Answer from the drawing. Dimensions are ordinates in mm from the lowest x, y and z of the part. A direction names the side the tool comes from. Give positions to 0.01 mm unless a question says otherwise; leave off trailing zeros. Loops run counter-clockwise (first coordinate to the right, second up) from the corner with the lowest first, then second, coordinate; pieces in that order, holes last. Notation, with made-up numbers: M 1,-24.75 L 13,-24.75 A32 ccw 13,4.25 Z; hole C -12.5,53.5 d6. An arc over 180 degrees is marked long. Use a Markdown table: item, result.
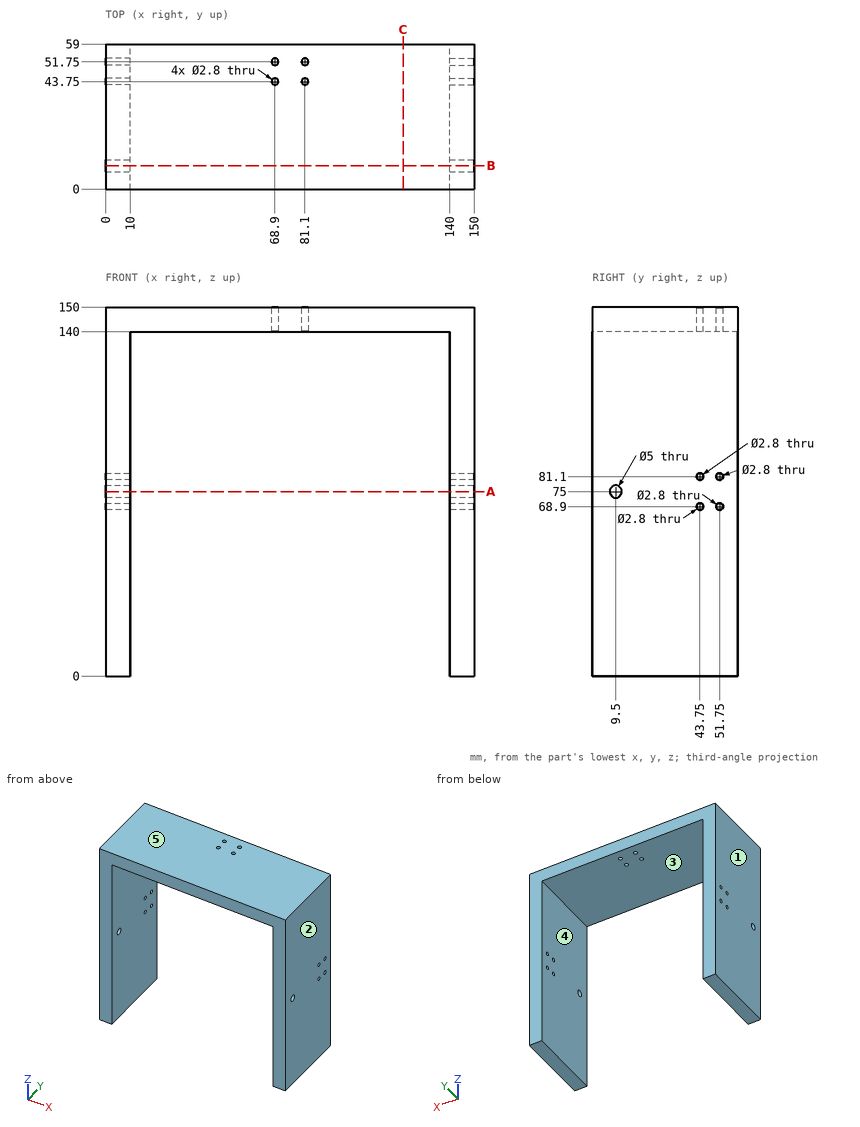
(1) A cutting plane is placed at B-B (y = 9.5). Write down the section's boundary in (x, z).
Entries:
| item | result |
|---|---|
| outline | M 0,0 L 10,0 L 10,72.5 L 0,72.5 Z; M 0,77.5 L 10,77.5 L 10,140 L 140,140 L 140,77.5 L 150,77.5 L 150,150 L 0,150 Z; M 140,0 L 150,0 L 150,72.5 L 140,72.5 Z |
(2) Which of the six approach directions +Z, -Z, +X, -X, +Y, -Y give full straight-line access (tool end or side, diameter ignored) to the marked faces 4 and 5?
Entries:
| item | result |
|---|---|
| face 4 | -Z, +Y, -Y |
| face 5 | +Z, +X, -X, +Y, -Y |
(3) The mould has two halves that part along X. Classify the marked faces 1, 2 and 3: released by +X, released by -X, zero draft, split by the parting line, or undercut.
Entries:
| item | result |
|---|---|
| face 1 | released by -X |
| face 2 | released by +X |
| face 3 | undercut |
(4) Consider probe 1 along X at (y, z) = (51, 114.5); probe 2 along Z at (x, y) = (6, 43); probe 3 along Y at (x, z) = (7.25, 75). Determine where each line is inside the solid, lowest interval first. Write a range as [from, to].
Entries:
| item | result |
|---|---|
| probe 1 | x = [0, 10], [140, 150] |
| probe 2 | z = [0, 67.72], [70.08, 79.92], [82.28, 150] |
| probe 3 | y = [0, 7], [12, 59] |
(5) Given P1, Ø1.5, axis at x = 24, y = 49.5, coming from the -Z side, flat-ended and moving along its own axis, determine where the tip first touches the part or whether it passes through.
Entries:
| item | result |
|---|---|
| P1 | stops at z = 140 |
(6) A cutting plane is placed at C-C (x = 121). Write down the section's boundary in (y, z), and give its area (3 significant figures).
Entries:
| item | result |
|---|---|
| outline | M 0,140 L 59,140 L 59,150 L 0,150 Z |
| area | 590 mm² |
(7) A cutting plane is placed at A-A (z = 75). Write down the section's boundary in (x, y), and give its area (3 significant figures).
Entries:
| item | result |
|---|---|
| outline | M 0,0 L 10,0 L 10,7 L 0,7 Z; M 0,12 L 10,12 L 10,59 L 0,59 Z; M 140,0 L 150,0 L 150,7 L 140,7 Z; M 140,12 L 150,12 L 150,59 L 140,59 Z |
| area | 1,080 mm² |
